from build123d import *

# Parameters (mm, degrees)
EXTRUDE_1_DEPTH             = 90
SKETCH_2_W                  = 90
SKETCH_2_H                  = 42.75
EXTRUDE_2_DEPTH             = 8.2
SKETCH_3_W                  = 90
SKETCH_3_H                  = 52.45
EXTRUDE_3_DEPTH             = 8.2
SKETCH_4_W                  = 3.95
SKETCH_4_H                  = 2.25
CUT_EXTRUDE_1_DEPTH         = 91
SKETCH_5_W                  = 3.95
SKETCH_5_H                  = 29.5
CUT_EXTRUDE_2_DEPTH         = 91
SKETCH_6_W                  = 3.95
SKETCH_6_H                  = 6.2
CUT_EXTRUDE_3_DEPTH         = 91
SKETCH_7_W                  = 2.25
SKETCH_7_H                  = 3.95
CUT_EXTRUDE_4_DEPTH         = 91
SKETCH_8_W                  = 4.5
SKETCH_8_H                  = 3.95
CUT_EXTRUDE_5_DEPTH         = 91
SKETCH_9_W                  = 9
SKETCH_9_H                  = 3.95
CUT_EXTRUDE_6_DEPTH         = 91
SKETCH_10_W                 = 4.5
SKETCH_10_H                 = 3.95
CUT_EXTRUDE_7_DEPTH         = 91
SKETCH_11_W                 = 2.25
SKETCH_11_H                 = 3.95
CUT_EXTRUDE_8_DEPTH         = 91
SKETCH_12_W                 = 46.1
SKETCH_12_H                 = 44.6
CUT_EXTRUDE_9_DEPTH         = 86.2
HOLE_WIZARD_2_5_2_5_1_D     = 2.5
HOLE_WIZARD_2_5_2_5_1_DEPTH = 90
HOLE_WIZARD_4_5_4_5_1_D     = 4.5
HOLE_WIZARD_4_5_4_5_1_DEPTH = 90
SKETCH_19_R                 = 1.67252853
SKETCH_19_R_2               = 1.459159852
SKETCH_19_R_3               = 1.459908976
SKETCH_19_R_4               = 1.592821911
SKETCH_19_R_5               = 1.532216665
SKETCH_19_R_6               = 1.596138091
EXTRUDE_4_DEPTH             = 90
FILLET_1_R                  = 2
FILLET_2_R                  = 2
FILLET_3_R                  = 2
FILLET_4_R                  = 2
FILLET_5_R                  = 2
FILLET_6_R                  = 2
FILLET_7_R                  = 2
FILLET_8_R                  = 2
FILLET_9_R                  = 2
FILLET_10_R                 = 2
FILLET_11_R                 = 2
FILLET_12_R                 = 2
EXTRUDE_5_DEPTH             = 0.4


with BuildPart() as part:
    # Эскиз1 → Бобышка-Вытянуть1 (new body)
    with BuildSketch(Plane(origin=(90, 0, 0), x_dir=(0, 0, -1), z_dir=(1, 0, 0))):
        with BuildLine():
            Line((6.75, 160.906238208), (6.75, 204.25))
            Line((6.75, 204.25), (-38.093761792, 204.25))
            ThreePointArc((-38.093761792, 204.25), (-41.825, 203), (-38.093761792, 201.75))
            Line((-38.093761792, 201.75), (-37.5, 201.75))
            Line((-37.5, 201.75), (-37.5, 168.25))
            Line((-37.5, 168.25), (-38.093761792, 168.25))
            ThreePointArc((-38.093761792, 168.25), (-41.825, 167), (-38.093761792, 165.75))
            Line((-38.093761792, 165.75), (-37.5, 165.75))
            Line((-37.5, 165.75), (-37.5, 161.5))
            Line((-37.5, 161.5), (-33.25, 161.5))
            Line((-33.25, 161.5), (-33.25, 160.906238208))
            ThreePointArc((-33.25, 160.906238208), (-32, 157.175), (-30.75, 160.906238208))
            Line((-30.75, 160.906238208), (-30.75, 161.5))
            Line((-30.75, 161.5), (-22.25, 161.5))
            Line((-22.25, 161.5), (-22.25, 160.906238208))
            ThreePointArc((-22.25, 160.906238208), (-21, 157.175), (-19.75, 160.906238208))
            Line((-19.75, 160.906238208), (-19.75, 161.5))
            Line((-19.75, 161.5), (-6.75, 161.5))
            Line((-6.75, 161.5), (-6.75, 160.906238208))
            ThreePointArc((-6.75, 160.906238208), (-5.5, 157.175), (-4.25, 160.906238208))
            Line((-4.25, 160.906238208), (-4.25, 161.5))
            Line((-4.25, 161.5), (4.25, 161.5))
            Line((4.25, 161.5), (4.25, 160.906238208))
            ThreePointArc((4.25, 160.906238208), (5.5, 157.175), (6.75, 160.906238208))
        make_face()
    extrude(amount=-EXTRUDE_1_DEPTH)

    # Эскиз2 → Бобышка-Вытянуть2 (add)
    with BuildSketch(Plane(origin=(0, 0, -6.75), x_dir=(-1, 0, 0), z_dir=(0, 0, -1))):
        with Locations((-45, 182.875)):
            Rectangle(SKETCH_2_W, SKETCH_2_H)
    extrude(amount=EXTRUDE_2_DEPTH)

    # Эскиз3 → Бобышка-Вытянуть3 (add)
    with BuildSketch(Plane(origin=(0, 204.25, 0), x_dir=(-1, 0, 0), z_dir=(0, 1, 0))):
        with Locations((-45, 11.275)):
            Rectangle(SKETCH_3_W, SKETCH_3_H)
    extrude(amount=EXTRUDE_3_DEPTH)

    # Эскиз4 → Вырез-Вытянуть1 (cut, through all)
    with BuildSketch(Plane.ZY):
        with Locations((-12.975, 162.625)):
            Rectangle(SKETCH_4_W, SKETCH_4_H)
    extrude(amount=-CUT_EXTRUDE_1_DEPTH, mode=Mode.SUBTRACT)

    # Эскиз5 → Вырез-Вытянуть2 (cut, through all)
    with BuildSketch(Plane.ZY):
        with Locations((-12.975, 185)):
            Rectangle(SKETCH_5_W, SKETCH_5_H)
    extrude(amount=-CUT_EXTRUDE_2_DEPTH, mode=Mode.SUBTRACT)

    # Эскиз6 → Вырез-Вытянуть3 (cut, through all)
    with BuildSketch(Plane.ZY):
        with Locations((-12.975, 209.35)):
            Rectangle(SKETCH_6_W, SKETCH_6_H)
    extrude(amount=-CUT_EXTRUDE_3_DEPTH, mode=Mode.SUBTRACT)

    # Эскиз7 → Вырез-Вытянуть4 (cut, through all)
    with BuildSketch(Plane.ZY):
        with Locations((-9.875, 210.475)):
            Rectangle(SKETCH_7_W, SKETCH_7_H)
    extrude(amount=-CUT_EXTRUDE_4_DEPTH, mode=Mode.SUBTRACT)

    # Эскиз8 → Вырез-Вытянуть5 (cut, through all)
    with BuildSketch(Plane.ZY):
        with Locations((0, 210.475)):
            Rectangle(SKETCH_8_W, SKETCH_8_H)
    extrude(amount=-CUT_EXTRUDE_5_DEPTH, mode=Mode.SUBTRACT)

    # Эскиз9 → Вырез-Вытянуть6 (cut, through all)
    with BuildSketch(Plane.ZY):
        with Locations((13.25, 210.475)):
            Rectangle(SKETCH_9_W, SKETCH_9_H)
    extrude(amount=-CUT_EXTRUDE_6_DEPTH, mode=Mode.SUBTRACT)

    # Эскиз10 → Вырез-Вытянуть7 (cut, through all)
    with BuildSketch(Plane.ZY):
        with Locations((26.5, 210.475)):
            Rectangle(SKETCH_10_W, SKETCH_10_H)
    extrude(amount=-CUT_EXTRUDE_7_DEPTH, mode=Mode.SUBTRACT)

    # Эскиз11 → Вырез-Вытянуть8 (cut, through all)
    with BuildSketch(Plane.ZY):
        with Locations((36.375, 210.475)):
            Rectangle(SKETCH_11_W, SKETCH_11_H)
    extrude(amount=-CUT_EXTRUDE_8_DEPTH, mode=Mode.SUBTRACT)

    # Эскиз12 → Вырез-Вытянуть9 (cut)
    with BuildSketch(Plane(origin=(90, 0, 0), x_dir=(0, 0, -1), z_dir=(1, 0, 0))):
        with Locations((-13.25, 185)):
            Rectangle(SKETCH_12_W, SKETCH_12_H)
    extrude(amount=-CUT_EXTRUDE_9_DEPTH, mode=Mode.SUBTRACT)

    # Диаметр отверстия Ø2.5 (2.5)1
    with Locations(Plane(origin=(90, 0, 0), x_dir=(0, 0, -1), z_dir=(1, 0, 0))):
        with Locations((5.5, 159.25), (-21, 159.25), (-5.5, 159.25), (-32, 159.25), (-39.75, 167), (-39.75, 203)):
            Hole(HOLE_WIZARD_2_5_2_5_1_D / 2, depth=HOLE_WIZARD_2_5_2_5_1_DEPTH)

    # Диаметр отверстия Ø4.5 (4.5)1
    with Locations(Plane.ZY):
        with Locations((-13.25, 167), (-13.25, 203), (-5.5, 210.75), (5.5, 210.75), (21, 210.75), (32, 210.75)):
            Hole(HOLE_WIZARD_4_5_4_5_1_D / 2, depth=HOLE_WIZARD_4_5_4_5_1_DEPTH)

    # Эскиз19 → Бобышка-Вытянуть4 (add)
    with BuildSketch(Plane(origin=(90, 0, 0), x_dir=(0, 0, -1), z_dir=(1, 0, 0))):
        with Locations((-39.75, 203)):
            Circle(SKETCH_19_R)
        with Locations((-39.75, 167)):
            Circle(SKETCH_19_R_2)
        with Locations((-32, 159.25)):
            Circle(SKETCH_19_R_3)
        with Locations((-21, 159.25)):
            Circle(SKETCH_19_R_4)
        with Locations((-5.5, 159.25)):
            Circle(SKETCH_19_R_5)
        with Locations((5.5, 159.25)):
            Circle(SKETCH_19_R_6)
    extrude(amount=-EXTRUDE_4_DEPTH)

    # Скругление1
    fillet_1_edges = [part.edges().sort_by_distance(p)[0] for p in [
        (45, 208.5, -8.75),
    ]]
    fillet(fillet_1_edges, radius=FILLET_1_R)

    # Скругление2
    fillet_2_edges = [part.edges().sort_by_distance(p)[0] for p in [
        (45, 163.75, -11),
    ]]
    fillet(fillet_2_edges, radius=FILLET_2_R)

    # Скругление3
    fillet_3_edges = [part.edges().sort_by_distance(p)[0] for p in [
        (45, 170.25, -11),
    ]]
    fillet(fillet_3_edges, radius=FILLET_3_R)

    # Скругление4
    fillet_4_edges = [part.edges().sort_by_distance(p)[0] for p in [
        (45, 199.75, -11),
    ]]
    fillet(fillet_4_edges, radius=FILLET_4_R)

    # Скругление5
    fillet_5_edges = [part.edges().sort_by_distance(p)[0] for p in [
        (45, 206.25, -11),
    ]]
    fillet(fillet_5_edges, radius=FILLET_5_R)

    # Скругление6
    fillet_6_edges = [part.edges().sort_by_distance(p)[0] for p in [
        (45, 208.5, -2.25),
    ]]
    fillet(fillet_6_edges, radius=FILLET_6_R)

    # Скругление7
    fillet_7_edges = [part.edges().sort_by_distance(p)[0] for p in [
        (45, 208.5, 2.25),
    ]]
    fillet(fillet_7_edges, radius=FILLET_7_R)

    # Скругление8
    fillet_8_edges = [part.edges().sort_by_distance(p)[0] for p in [
        (45, 208.5, 8.75),
    ]]
    fillet(fillet_8_edges, radius=FILLET_8_R)

    # Скругление9
    fillet_9_edges = [part.edges().sort_by_distance(p)[0] for p in [
        (45, 208.5, 17.75),
    ]]
    fillet(fillet_9_edges, radius=FILLET_9_R)

    # Скругление10
    fillet_10_edges = [part.edges().sort_by_distance(p)[0] for p in [
        (45, 208.5, 24.25),
    ]]
    fillet(fillet_10_edges, radius=FILLET_10_R)

    # Скругление11
    fillet_11_edges = [part.edges().sort_by_distance(p)[0] for p in [
        (45, 208.5, 28.75),
    ]]
    fillet(fillet_11_edges, radius=FILLET_11_R)

    # Скругление12
    fillet_12_edges = [part.edges().sort_by_distance(p)[0] for p in [
        (45, 208.5, 35.25),
    ]]
    fillet(fillet_12_edges, radius=FILLET_12_R)

    # Эскиз21 → Бобышка-Вытянуть5 (add)
    with BuildSketch(Plane.ZY):
        with BuildLine():
            Line((-11, 192.615858601), (4.026059703, 212.45))
            ThreePointArc((4.026059703, 212.45), (-19.762874791, 214.863320113), (-11, 192.615858601))
        make_face()
        with BuildLine():
            Line((22.473940297, 212.45), (37.5, 192.207288754))
            ThreePointArc((37.5, 192.207288754), (46.120046397, 214.304143308), (22.473940297, 212.45))
        make_face()
        with BuildLine():
            Line((37.5, 177.792711246), (22.473940297, 157.55))
            ThreePointArc((22.473940297, 157.55), (46.120046397, 155.695856692), (37.5, 177.792711246))
        make_face()
        with BuildLine():
            Line((4.026059703, 157.55), (-11, 177.384141399))
            ThreePointArc((-11, 177.384141399), (-19.762874791, 155.136679887), (4.026059703, 157.55))
        make_face()
    extrude(amount=-EXTRUDE_5_DEPTH)


solid = part.part
Verification items for the finished model (mm, model axes). A direction names the side the tool comes from. Give positions to 0.01 mm unless a question says otherwise; leave off trailing zeros. Order: outer loops, then holes, each group sorted by start corner. A loop starts at its lowest first (then second) coordinate and runs counter-clockwise, first axis right, second up. Notation, with made-up numbers: (44.25, -9) -> (83.25, -9) arc R16 cw to (83.25, 5) -> close; hole circle Ø7 at (-11.75, 78.5). An arc over 180 degrees is marked (long way). Answer as CSV lines item,"result".
Q1. Depth check by flat-ended pin: pin 1 (1.5 mm diameter, centred on y = 212, z = 37, fed in from +X); pin 2 (8 mm diameter, centred on x = 11, y = 190.5, fed in from +Z); pin 3 (2 mm diameter, centred on x = 47.5, z = -14, fed in from -Y). Enter the tip coordinate at first touch or a pass-through.
Solutions:
pin 1,"stops at x = 0.4"
pin 2,"stops at z = 37.5"
pin 3,"stops at y = 163.75"
Q2. Sectioned sample at B-B on y = 159.25. Record the cut outline in (x, z) (3 decimals).
Solutions:
outline,"(0, -21.914) -> (0.4, -21.914) -> (0.4, -7.575) -> (90, -7.575) -> (90, -3.425) -> (0.4, -3.425) -> (0.4, 2.738) -> (0, 2.738) -> close; (0, 3.425) -> (90, 3.425) -> (90, 7.575) -> (0, 7.575) -> close; (0, 18.925) -> (90, 18.925) -> (90, 23.075) -> (0, 23.075) -> close; (0, 23.736) -> (0.4, 23.736) -> (0.4, 29.925) -> (90, 29.925) -> (90, 34.075) -> (0.4, 34.075) -> (0.4, 48.034) -> (0, 48.034) -> close"
Q3. Release check for a two-part mould opening along Z. For faces 4 (the flat face through (90, 162, 11)), 5 (the cylindrical face through (0.2, 215.2, -19.5)), 6 (the flat face through (44, 185, -11)) record: +Z half, -Z half, draft (parallel to the pull), parting line (faces both ways), or undercut.
Solutions:
face 4,"draft"
face 5,"undercut"
face 6,"-Z half"
Q4. Sectioned sample at C-C on z = 39.75. Record the cut outline in (x, y) (3 decimals), plus the area to 3 significant figures.
Solutions:
outline,"(0, 150.915) -> (0.4, 150.915) -> (0.4, 164.925) -> (90, 164.925) -> (90, 169.075) -> (0.4, 169.075) -> (0.4, 177.165) -> (0, 177.165) -> close; (0, 192.835) -> (0.4, 192.835) -> (0.4, 200.925) -> (90, 200.925) -> (90, 205.075) -> (0.4, 205.075) -> (0.4, 219.085) -> (0, 219.085) -> close"
area,"765 mm²"
Q5. Access from +Z, -Z, +X, -X, +Y, -Y to the whole of each face (thin tool, end or side, straight path). Record for faces 1 (the cylindrical face through (45.83, 208.5, -5.42)), 2 (the flat face through (44, 208.5, 13)), 3 (the flat face through (46, 164, 37.5)).
Solutions:
face 1,"+X"
face 2,"+X, -X, +Y"
face 3,"+X, -Y"
Q6. Sectioned sample at A-A on z = 5.5. Record the cut outline in (x, y) (3 decimals).
Solutions:
outline,"(0, 157.175) -> (90, 157.175) -> (90, 162.7) -> (3.8, 162.7) -> (3.8, 207.3) -> (90, 207.3) -> (90, 208.5) -> (0, 208.5) -> close"
Q7. Sectioned sample at D-D on y = 203. Record the cut outline in (x, z) (3 decimals), plus the area to 3 significant figures.
Solutions:
outline,"(0, -22.182) -> (0.4, -22.182) -> (0.4, -11) -> (90, -11) -> (90, -9.8) -> (3.8, -9.8) -> (3.8, 36.3) -> (90, 36.3) -> (90, 41.825) -> (0.4, 41.825) -> (0.4, 48.562) -> (0, 48.562) -> close"
area,"788 mm²"
Q8. Scan lines: probe 1 along Y at (x, z) = (68, -13.25); probe 2 along Z at (x, y) = (58, 181.5); probe 3 along Y at (x, z) = (11.5, 3). Record each from-to range of solid material in increasing order.
Solutions:
probe 1,"y = 163.75 to 164.75, 169.25 to 170.25, 199.75 to 200.75, 205.25 to 206.25"
probe 2,"z = -11 to -9.8, 36.3 to 37.5"
probe 3,"y = 161.5 to 162.7, 207.3 to 212.45"
